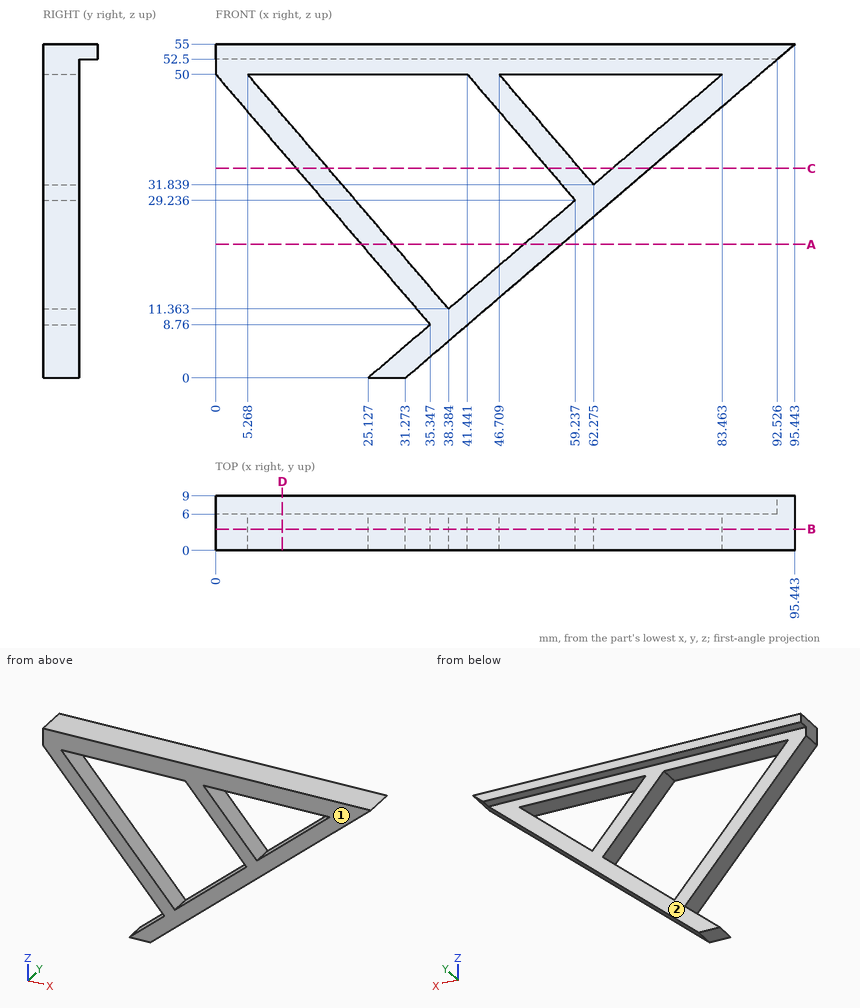
For this review, use the dimensioned drawing (mm, ordinates from the lowest corner) and the shaded views. A direction names the side the tool comes from. Round coordinates to 2 decimals unless told otherwise and drop trailing zeros. Order: outer loops, then holes, each group sorted by start corner. A loop starts at its lowest first (then second) coordinate and runs counter-clockwise, first axis right, second up. Notation, with made-up numbers: (-19, -12.5) -> (0, -12.5) arc R19 cw to (0, 21.5) -> close; hole circle Ø4 at (30.5, 67.25). An arc over 180 degrees is marked (long way). Write item = value, one per line. Start each with the question number.
Item 1: For line 1 along X through (y, z) = (5, 35) (1 decimal); line 2 along Z through (x, y) = (47.5, 3.25) (1 decimal); line 3 along Z through (x, y) = (67, 8.5), list the stretches that pass through material, from the lowest coordinate up.
Item 2: For the marked faces 1 and 2, list the 3-axis set-ups (+Z, -Z, +X, -X, +Y, -Y) from which the entire face can be reached by the end or side of a thin tool; tool diameter is ignored.
Item 3: Consider section B-B on y = 3.5. Write out the cut boundary in (x, z) (1 decimal), plus the area to 3 significant figures.
Item 4: Consider section A-A on z = 22. Write out the cut boundary in (x, y) (1 decimal).
Item 5: Clearance check with flat-ended pins moving along their axes: pin 1 Ø3 at (x, y) = (61, 4.5) entering from -Z; pin 2 Ø2 at (y, z) = (1, 30) entering from -X (1 decimal); pin 3 Ø5 at (y, z) = (2, 27) entering from +X. State where each tip first meets the part, or that it passes through.
Item 6: Consider section C-C on z = 34.5. Write out the cut boundary in (x, y) (1 decimal), plus the area to 3 significant figures.
Item 7: Consider section D-D on x = 11. Write out the cut boundary in (y, z).
Conclusion:
q1.line_1 = 12.9 to 18.1, 54.3 to 59.6, 66 to 72.1
q1.line_2 = 13.9 to 19.2, 42.9 to 49.1, 50 to 55
q1.line_3 = 52.5 to 55
q2.face_1 = +Z, -Z, +X, -X, -Y
q2.face_2 = -Z, +X, -X, +Y
q3.outline = (0, 50) -> (35.3, 8.8) -> (25.1, 0) -> (31.3, 0) -> (95.4, 55) -> (0, 55) -> close; hole (5.3, 50) -> (38.4, 11.4) -> (59.2, 29.2) -> (41.4, 50) -> close; hole (46.7, 50) -> (62.3, 31.8) -> (83.5, 50) -> close
q3.area = 1,080 mm2
q4.outline = (24, 0) -> (29.3, 0) -> (29.3, 6) -> (24, 6) -> close; (50.8, 0) -> (56.9, 0) -> (56.9, 6) -> (50.8, 6) -> close
q5.pin_1 = 24.19
q5.pin_2 = 16.3
q5.pin_3 = 65.69
q6.outline = (13.3, 0) -> (18.6, 0) -> (18.6, 6) -> (13.3, 6) -> close; (54.7, 0) -> (60, 0) -> (60, 6) -> (54.7, 6) -> close; (65.4, 0) -> (71.5, 0) -> (71.5, 6) -> (65.4, 6) -> close
q6.area = 100 mm2
q7.outline = (0, 37.17) -> (6, 37.17) -> (6, 43.31) -> (0, 43.31) -> close; (0, 50) -> (6, 50) -> (6, 52.5) -> (9, 52.5) -> (9, 55) -> (0, 55) -> close
